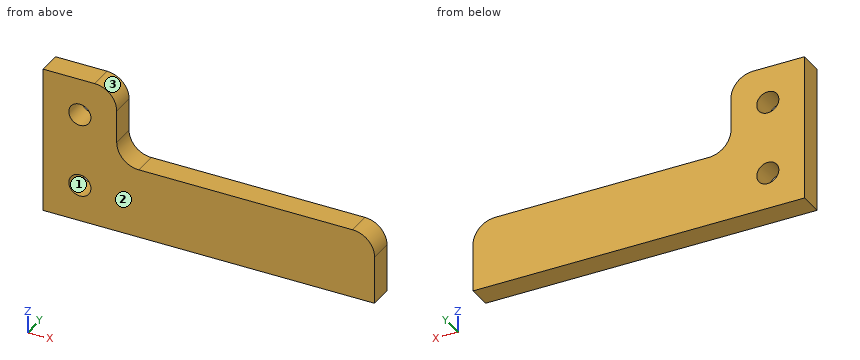
from build123d import *

# Parameters (mm, degrees)
BOSS_EXTRUDE1_DEPTH          = 3.175
F_3_0_3_DIAMETER_HOLE1_D     = 3
F_3_0_3_DIAMETER_HOLE1_DEPTH = 10
F_3_0_3_DIAMETER_HOLE1_TIP   = 0.901290929


with BuildPart() as part:
    # Sketch1 → Boss-Extrude1 (new body)
    with BuildSketch(Plane(origin=(0, 0, 0), x_dir=(1, 0, 0), z_dir=(0, 1, 0))):
        with BuildLine():
            Line((0, 0), (45, 0))
            Line((45, 0), (45, -6.539392014))
            ThreePointArc((45, -6.539392014), (44.121320344, -8.660712358), (42, -9.539392014))
            Line((42, -9.539392014), (13, -9.539392014))
            ThreePointArc((13, -9.539392014), (10.878679656, -10.418071671), (10, -12.539392014))
            Line((10, -12.539392014), (10, -17))
            ThreePointArc((10, -17), (9.121320344, -19.121320344), (7, -20))
            Line((7, -20), (0, -20))
            Line((0, -20), (0, 0))
        make_face()
    extrude(amount=BOSS_EXTRUDE1_DEPTH)

    # Ø3.0 (3) Diameter Hole1
    with Locations(Plane(origin=(0, 3.175, 0), x_dir=(-1, 0, 0), z_dir=(0, 1, 0))):
        with Locations((-5, 5), (-5, 15)):
            Hole(F_3_0_3_DIAMETER_HOLE1_D / 2, depth=F_3_0_3_DIAMETER_HOLE1_DEPTH)
            with Locations((0, 0, -(F_3_0_3_DIAMETER_HOLE1_DEPTH + F_3_0_3_DIAMETER_HOLE1_TIP / 2))):  # 118° drill point
                Cone(0, F_3_0_3_DIAMETER_HOLE1_D / 2, F_3_0_3_DIAMETER_HOLE1_TIP, mode=Mode.SUBTRACT)


solid = part.part
Geometry check sheet. Reference: the model listing, model coordinates, mm. Face numbers are marked on the shaded views. Coordinates: 2 decimals unless noted, no trailing zeros. Loops run counter-clockwise (first coordinate to the right, second up) from the corner with the lowest first, then second, coordinate; pieces in that order, holes last. Notation, with made-up numbers: (1.5, 74) - (43.5, 74) arc R29 cw to (43.5, 113) - close; hole circle Ø1 at (-17, -5.5). An arc over 180 degrees is marked (long way). Use one line per item in the form item = value. Start each with the question number.
Item 1: Section check C-C, the plane y = 1.55. Enter the section's corners in (x, z), and give its area (3 significant figures).
Item 2: Section check B-B, the plane x = 5. Enter the section's corners in (y, z) (3 decimals), and give its area (4 significant figures).
Item 3: Mould release check, pull along Z, two halves, no side actions. Record for the marked faces 1, 2 and 3: +Z half, -Z half, draft (parallel to the pull), parting line (faces both ways), or undercut.
Item 4: Thickness scan on probe 1 along Z at (x, y) = (5, 1.5); probe 2 along Z at (x, y) = (20.5, 1.25); probe 3 along X at (y, z) = (1.65, 6). Record the ranges inside material, lowest first.
Item 5: Section check D-D, the plane z = 15. Enter the section's corners in (x, y) (3 decimals), and give its area (3 significant figures).
Item 6: Gauge pin test, flat ends, axial feed: pin 1 (1 mm diameter, centred on x = 33, y = 0.5, fed in from +Z); pin 2 (1.6 mm diameter, centred on y = 1.5, z = 14.5, fed in from +X). Record the tip position at first contact, or that the pin passes through.
Item 7: Section check A-A, the plane z = 5. Enter the section's corners in (x, y) (3 decimals), and give its area (3 significant figures).
Computed:
q1.outline = (0, 0) - (45, 0) - (45, 6.54) arc R3 ccw to (42, 9.54) - (13, 9.54) arc R3 cw to (10, 12.54) - (10, 17) arc R3 ccw to (7, 20) - (0, 20) - close; hole circle Ø3 at (5, 5); hole circle Ø3 at (5, 15)
q1.area = 518 mm2
q2.outline = (0, 0) - (3.175, 0) - (3.175, 3.5) - (0, 3.5) - close; (0, 6.5) - (3.175, 6.5) - (3.175, 13.5) - (0, 13.5) - close; (0, 16.5) - (3.175, 16.5) - (3.175, 20) - (0, 20) - close
q2.area = 44.45 mm2
q3.face_1 = undercut
q3.face_2 = draft
q3.face_3 = +Z half
q4.probe_1 = 0 to 3.5, 6.5 to 13.5, 16.5 to 20
q4.probe_2 = 0 to 9.54
q4.probe_3 = 0 to 3.88, 6.12 to 45
q5.outline = (0, 0) - (3.5, 0) - (3.5, 3.175) - (0, 3.175) - close; (6.5, 0) - (10, 0) - (10, 3.175) - (6.5, 3.175) - close
q5.area = 22.2 mm2
q6.pin_1 = 9.54
q6.pin_2 = 10
q7.outline = (0, 0) - (3.5, 0) - (3.5, 3.175) - (0, 3.175) - close; (6.5, 0) - (45, 0) - (45, 3.175) - (6.5, 3.175) - close
q7.area = 133 mm2
